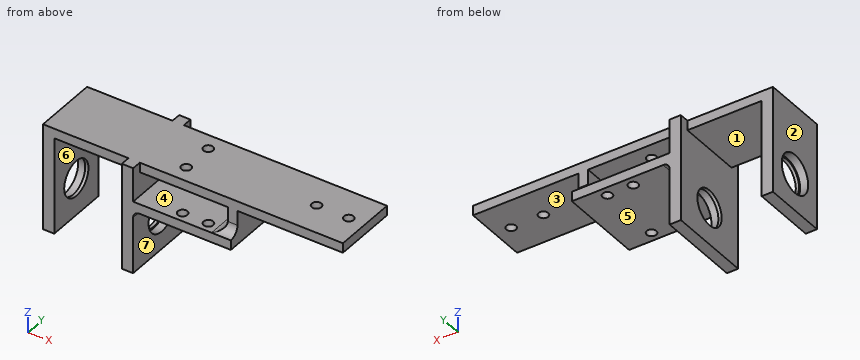
from build123d import *

# Parameters (mm, degrees)
SKETCH_1_W          = 20
SKETCH_1_H          = 20
SKETCH_1_R          = 1.5
SKETCH_1_W_2        = 23
SKETCH_1_W_3        = 3.5
EXTRUDE_1_DEPTH     = 3
EXTRUDE_2_DEPTH     = 30
SKETCH_1_4_W        = 3.5
SKETCH_1_4_H        = 20
EXTRUDE_3_DEPTH     = 30
SKETCH_3_R          = 6
CUT_EXTRUDE_2_DEPTH = 38
SKETCH_4_R          = 6
SKETCH_4_R_2        = 5.5
EXTRUDE_4_DEPTH     = 1
EXTRUDE_START       = -1
SKETCH_5_R          = 6
SKETCH_5_R_2        = 5.5
EXTRUDE_5_DEPTH     = 1
SKETCH_7_R          = 1.5
CUT_EXTRUDE_4_DEPTH = 5
SKETCH_9_W          = 3
SKETCH_9_H          = 26
EXTRUDE_6_DEPTH     = 30.3
SKETCH_10_R         = 1.5
CUT_EXTRUDE_6_DEPTH = 10
FILLET_2_R          = 2
SKETCH_13_W         = 3
SKETCH_13_H         = 20
EXTRUDE_8_DEPTH     = 10.5
FILLET_5_R          = 3


with BuildPart() as part:
    # 草图1 → 凸台-拉伸1 (new body)
    # profile 1 of 5: a face of its own
    with BuildSketch(Plane.XY):
        Polygon((-10, -10.145751311), (-10, 9.854248689), (-53, 9.854248689), (-53, -0.145751311), (-53, -10.145751311), align=None)
    # profile 2 of 5: a face of its own
    with BuildSketch(Plane.XY):
        with Locations((0, -0.145751311)):
            Rectangle(SKETCH_1_W, SKETCH_1_H)
        with Locations((-5, -0.145751311)):
            Circle(SKETCH_1_R, mode=Mode.SUBTRACT)
        with Locations((5, -0.145751311)):
            Circle(SKETCH_1_R, mode=Mode.SUBTRACT)
    # profile 3 of 5: a face of its own
    with BuildSketch(Plane.XY):
        Polygon((-53, -0.145751311), (-53, 9.854248689), (-53, 12.854248689), (-56.5, 12.854248689), (-56.5, 9.854248689), (-56.5, -10.145751311), (-56.5, -13.145751311), (-53, -13.145751311), (-53, -10.145751311), align=None)
    # profile 4 of 5: a face of its own
    with BuildSketch(Plane.XY):
        with Locations((-68, -0.145751311)):
            Rectangle(SKETCH_1_W_2, SKETCH_1_H)
    # profile 5 of 5: a face of its own
    with BuildSketch(Plane.XY):
        with Locations((-81.25, -0.145751311)):
            Rectangle(SKETCH_1_W_3, SKETCH_1_H)
    extrude(amount=EXTRUDE_1_DEPTH)

    # 草图1<3> → 凸台-拉伸2 (add)
    with BuildSketch(Plane.XY):
        Polygon((-53, -0.145751311), (-53, 9.854248689), (-53, 12.854248689), (-56.5, 12.854248689), (-56.5, 9.854248689), (-56.5, -10.145751311), (-56.5, -13.145751311), (-53, -13.145751311), (-53, -10.145751311), align=None)
    extrude(amount=-EXTRUDE_2_DEPTH)

    # 草图1<4> → 凸台-拉伸3 (add)
    with BuildSketch(Plane.XY):
        with Locations((-81.25, -0.145751311)):
            Rectangle(SKETCH_1_4_W, SKETCH_1_4_H)
    extrude(amount=-EXTRUDE_3_DEPTH)

    # 草图3 → 切除-拉伸2 (cut)
    with BuildSketch(Plane.ZY.offset(83)):
        with Locations((-18.5, -0.145751311)):
            Circle(SKETCH_3_R)
    extrude(amount=-CUT_EXTRUDE_2_DEPTH, mode=Mode.SUBTRACT)

    # 草图4 → 凸台-拉伸4 (add)
    with BuildSketch(Plane.ZY.offset(56.5)):
        with Locations((-18.5, -0.145751311)):
            Circle(SKETCH_4_R)
        with Locations((-18.5, -0.145751311)):
            Circle(SKETCH_4_R_2, mode=Mode.SUBTRACT)
    extrude(amount=-EXTRUDE_4_DEPTH)

    # 草图5 → 凸台-拉伸5 (add)
    with BuildSketch(Plane(origin=(-79.5, 0, 0), x_dir=(0, 0, -1), z_dir=(1, 0, 0)).offset(EXTRUDE_START)):
        with Locations(Location((18.5, -0.145751311, 0), (0, 0, 180))):
            Circle(SKETCH_5_R)
        with Locations(Location((18.5, -0.145751311, 0), (0, 0, 180))):
            Circle(SKETCH_5_R_2, mode=Mode.SUBTRACT)
    extrude(amount=EXTRUDE_5_DEPTH)

    # 草图7 → 切除-拉伸4 (cut)
    with BuildSketch(Plane.XY.offset(3)):
        with Locations((-42, 4.853948946)):
            Circle(SKETCH_7_R)
        with Locations((-42, -5.146051054)):
            Circle(SKETCH_7_R)
    extrude(amount=-CUT_EXTRUDE_4_DEPTH, mode=Mode.SUBTRACT)

    # 草图9 → 凸台-拉伸6 (add)
    with BuildSketch(Plane(origin=(-53, 0, 0), x_dir=(0, 0, -1), z_dir=(1, 0, 0))):
        with Locations((9, -0.145751311)):
            Rectangle(SKETCH_9_W, SKETCH_9_H)
    extrude(amount=EXTRUDE_6_DEPTH)

    # 草图10 → 切除-拉伸6 (cut)
    with BuildSketch(Plane.XY.offset(-7.5)):
        with Locations((-31.699132707, 9.854844931)):
            Circle(SKETCH_10_R)
        with Locations((-39.699132705, 9.855007549)):
            Circle(SKETCH_10_R)
        with Locations((-31.699403758, -10.146618604)):
            Circle(SKETCH_10_R)
        with Locations((-39.699403758, -10.146618604)):
            Circle(SKETCH_10_R)
    extrude(amount=-CUT_EXTRUDE_6_DEPTH, mode=Mode.SUBTRACT)

    # 圆角2
    fillet_2_edges = [part.edges().sort_by_distance(p)[0] for p in [
        (-53, -0.145751311, -10.5),
    ]]
    fillet(fillet_2_edges, radius=FILLET_2_R - 0.0001)  # a hair under: the kernel refuses the full size

    # 草图13 → 凸台-拉伸8 (add)
    with BuildSketch(Plane(origin=(0, 0, -10.5), x_dir=(-1, 0, 0), z_dir=(0, 0, -1))):
        with Locations((24.2, -0.145751311)):
            Rectangle(SKETCH_13_W, SKETCH_13_H)
    extrude(amount=-EXTRUDE_8_DEPTH)

    # 圆角5
    fillet_5_edges = [part.edges().sort_by_distance(p)[0] for p in [
        (-24.2, 9.854248689, -7.5),
        (-25.7, -0.145751311, -7.5),
        (-24.2, -10.145751311, -7.5),
    ]]
    fillet(fillet_5_edges, radius=FILLET_5_R - 0.0001)  # a hair under: the kernel refuses the full size


solid = part.part
For this review, take the finished solid that the model builds, in its own axes (mm). Face numbers are marked on the shaded views. A direction names the side the tool comes from. Give positions to 0.01 mm unless a question says otherwise; leave off trailing zeros. Loops run counter-clockwise (first coordinate to the right, second up) from the corner with the lowest first, then second, coordinate; pieces in that order, holes last. Notation, with made-up numbers: M 33,85.5 L 60,85.5 A14 cw 60,90.5 Z; hole C -0.5,32 d5. An arc over 180 degrees is marked long. Put each result on its own line as item: value. Start each with the question number.
(1) Add section A-A, the plane z = -25.5. Write out the cut boundary in (x, y).
(2) Add section C-C, the plane z = -18.5. Write out the cut boundary in (x, y).
(3) Add section B-B, the plane x = -49. Write out the cut boundary in (y, z), then the cut area to 3 significant figures.
(4) Wall thickness on L1, parallel to Y at x = -42, z = 1; L2, parallel to X at y = -5.5, z = -24; L3, parallel to X at y = -0.75, z = -2: over which ranges is each line inside the solid? List them lowest first.
(5) The part is to be moulded in two halves that separate along X. For the marked faces 5, 6 and 7, say which applies: +X half, -X half, draft (parallel to the pull), parting line (faces both ways), or undercut.
(6) Machinability: for the marked faces 1, 2, 3 and 4, which of the approach directions +Z, -Z, +X, -X, +Y, -Y give a long, thin tool a straight path to every point of the face, cutting with its end or side? Answer none if there is none.
(7) For pin 1 (9.5 mm diameter, centred on y = 2.5, z = -18.5, fed in from +X); pin 2 (1.8 mm diameter, centred on x = -42, y = -5.15, fed in from -Z); pin 3 (5 mm diameter, centred on y = -2.5, z = -6, fed in from +X); pin 4 (7 mm diameter, centred on y = -0.15, z = -18.5, fed in from -X), all flat-tipped, find the tip position at first contact; note any pin that passes through.
(8) Add section D-D, the plane x = 2.5. Write out the cut boundary in (y, z).
Result:
1. outline: M -83,-10.15 L -79.5,-10.15 L -79.5,9.85 L -83,9.85 Z; M -56.5,-13.15 L -53,-13.15 L -53,12.85 L -56.5,12.85 Z
2. outline: M -83,-10.15 L -79.5,-10.15 L -79.5,-5.65 L -80.5,-5.65 L -80.5,-6.15 L -83,-6.15 Z; M -83,5.85 L -80.5,5.85 L -80.5,5.35 L -79.5,5.35 L -79.5,9.85 L -83,9.85 Z; M -56.5,-13.15 L -53,-13.15 L -53,-6.15 L -55.5,-6.15 L -55.5,-5.65 L -56.5,-5.65 Z; M -56.5,5.35 L -55.5,5.35 L -55.5,5.85 L -53,5.85 L -53,12.85 L -56.5,12.85 Z
3. outline: M -13.15,-10.5 L 12.85,-10.5 L 12.85,-7.5 L -13.15,-7.5 Z; M -10.15,0 L 9.85,0 L 9.85,3 L -10.15,3 Z
3. area: 138 mm^2
4. L1: y = -10.15 to -6.65, -3.65 to 3.35, 6.35 to 9.85
4. L2: x = -83 to -79.5, -56.5 to -53
4. L3: x = -83 to -79.5, -56.5 to -53, -25.7 to -22.7
5. face 5: draft
5. face 6: undercut
5. face 7: +X half
6. face 1: -Z, +Y, -Y
6. face 2: +Z, -Z, -X, +Y, -Y
6. face 3: -Z, +X, +Y, -Y
6. face 4: +Y, -Y
7. pin 1: stops at x = -53
7. pin 2: stops at z = -10.5
7. pin 3: stops at x = -22.7
7. pin 4: passes through
8. outline: M -10.15,0 L 9.85,0 L 9.85,3 L -10.15,3 Z
